Can you work these out from the model? Positions are in its coordinate system, mm. A direction names the side the tool comes from. Coordinates: 2 decimals unless noted, no trailing zeros. Order: outer loops, then holes, each group sorted by start corner. A loop starts at its lowest first (then second) coordinate and runs counter-clockwise, first axis right, second up. Notation, with made-up numbers: (62, 43) - (109, 43) arc R26 cw to (109, 57) - close; hole circle Ø5 at (55, 73). An arc over 180 degrees is marked (long way). Use a Markdown table: item, result. Add a question column.
(1) For pin 1 Ø8 at (y, z) = (-38.5, -26) entering from +X; pin 2 Ø12 at (y, z) = (164, 72) entering from -X; pin 3 Ø2 at (x, y) = (49.5, -229) entering from +Z; pin 4 Ø1 at (y, z) = (-386, 62.5) entering from -X, each with a flat end and sliding along its axis, tell me the tip position at first contact or that it passes through.
(2) If I drill on L1, parallel to Z at x = 22.5, y = 290; L2, parallel to Y at x = 75.5, z = -91; L3, parallel to Z at x = 38, y = -435, over which ranges is the centre line in solid material (lowest first)? Write a range as [from, to].
(3) On a 3-axis mill with a long thin cutter (end or side, diameter ignored), from which of +Z, -Z, +X, -X, +Y, -Y can I reach the whole of each face in a straight line? I mean faces 1 (the flat face through (113, -22, 63.256)), 2 (the flat face through (113, 278, -32.859)), 3 (the flat face through (121, -572, -208.945)). Say none if no direction works.
(4) I want a section at B-B (y = 150). List the corners of the cut face in (x, z) for me.
(5) I want a section at D-D (z = -225). List the corners of the cut face in (x, y) for me, and give its area (3 significant figures).
(6) I want a section at C-C (x = 72). List the corners of the cut face in (y, z) for me, and give its area (3 significant figures).
(7) I want a section at A-A (z = -100.5). List the corners of the cut face in (x, y) for me.
(8) We'd pull the mould along Z, two halves only. Please class faces 4 (the flat face through (113, 284, -173.314)), 5 (the cylindrical face through (121.13, -568.75, 65.37)), 6 (the flat face through (113, 444.109, 15)), 7 (the flat face through (113, 225, -274.596)): pulls with the +Z half, pulls with the -Z half, needs draft (parallel to the pull), parting line crosses it, or undercut.
```python
from build123d import *

# Parameters (mm, degrees)
F0_W      = 1114.6509647369
F0_H      = 96.1142629385
F1_DEPTH  = 228.5858858377
F2_W      = 117.198035121
F2_H      = 274.5957672596
F3_DEPTH  = 229.3333578855
F4_W      = 229.3333578855
F4_H      = 456.3540816307
F5_DEPTH  = 101.281305775
F6_W      = 189.0553534031
F6_H      = 433.8834732771
F7_DEPTH  = 245.6944454461
F8_R      = 96.273971764
F9_DEPTH  = 484.469877556
F11_D     = 12.7
F11_DEPTH = 12.7
F11_TIP   = 3.8154649308


with BuildPart() as f1:
    # F0 (on Right) → F1 (new body)
    with BuildSketch(Plane.YZ):
        with Locations((-113.2168769836, 15.1985660195)):
            Rectangle(F0_W, F0_H)
    extrude(amount=F1_DEPTH)

    # F2 (on Right) → F3 (join)
    with BuildSketch(Plane.YZ):
        with Locations((58.5990175605, -137.2978836298)):
            Rectangle(F2_W, F2_H)
    extrude(amount=F3_DEPTH)

    # F4 (on face) → F5 (join)
    with BuildSketch(Plane(origin=(0, 0, -274.5957672596), x_dir=(1, 0, 0), z_dir=(0, 0, -1))):
        with Locations((114.6666789427, -228.1770408154)):
            Rectangle(F4_W, F4_H)
    extrude(amount=-F5_DEPTH)

    # F6 (on Right) → F7 (join)
    with BuildSketch(Plane.YZ):
        with Locations((-570.4715698957, 7.9966709018)):
            Rectangle(F6_W, F6_H)
    extrude(amount=F7_DEPTH)

    # F8 (on face) → F9 (cut)
    with BuildSketch(Plane(origin=(0, 0, 0), x_dir=(0, -1, 0), z_dir=(-1, 0, 0))):
        with Locations((664.9992465973, 63.2556974888)):
            Circle(F8_R)
    extrude(amount=-F9_DEPTH, mode=Mode.SUBTRACT)

    # F11
    with Locations(Plane(origin=(0, 0, -274.5957672596), x_dir=(1, 0, 0), z_dir=(0, 0, -1))):
        with Locations((107.4657961726, -350.3691852093)):
            Hole(F11_D / 2, depth=F11_DEPTH)
            with Locations((0, 0, -(F11_DEPTH + F11_TIP / 2))):  # 118° drill point
                Cone(0, F11_D / 2, F11_TIP, mode=Mode.SUBTRACT)


solid = f1.part
```
Answers follow:
| question | item | result |
|---|---|---|
| 1 | pin 1 | stops at x = 228.59 |
| 1 | pin 2 | passes through |
| 1 | pin 3 | stops at z = 63.26 |
| 1 | pin 4 | stops at x = 0 |
| 2 | L1 | z = [-274.6, -173.31], [-32.86, 63.26] |
| 2 | L2 | y = [-665, -475.94], [0, 117.2] |
| 2 | L3 | z = [-32.86, 63.26] |
| 3 | face 1 | +Z, +X, -X, +Y |
| 3 | face 2 | +X, -X, +Y |
| 3 | face 3 | -Z, +X, -X, -Y |
| 4 | outline | (0, -274.6) - (229.33, -274.6) - (229.33, -173.31) - (0, -173.31) - close; (0, -32.86) - (228.59, -32.86) - (228.59, 63.26) - (0, 63.26) - close |
| 5 | outline | (0, 0) - (229.33, 0) - (229.33, 456.35) - (0, 456.35) - close |
| 5 | area | 105,000 mm² |
| 6 | outline | (-665, -208.95) - (-475.94, -208.95) - (-475.94, -32.86) - (0, -32.86) - (0, -274.6) - (456.35, -274.6) - (456.35, -173.31) - (117.2, -173.31) - (117.2, -32.86) - (444.11, -32.86) - (444.11, 63.26) - (-475.94, 63.26) - (-475.94, 224.94) - (-665, 224.94) - (-665, 159.53) arc R96.27 cw to (-665, -33.02) - close |
| 6 | area | 219,000 mm² |
| 7 | outline | (0, -665) - (245.69, -665) - (245.69, -475.94) - (0, -475.94) - close; (0, 0) - (229.33, 0) - (229.33, 117.2) - (0, 117.2) - close |
| 8 | face 4 | undercut |
| 8 | face 5 | undercut |
| 8 | face 6 | needs draft |
| 8 | face 7 | pulls with the -Z half |
